from build123d import *

# Parameters (mm, degrees)
SKETCH1_R                = 5
BOSS_EXTRUDE1_DEPTH      = 120
SKETCH2_R                = 2.5
CUT_EXTRUDE1_DEPTH       = 20
SKETCH3_R                = 3
CUT_EXTRUDE2_DEPTH       = 80
SKETCH4_R                = 2
BOSS_EXTRUDE2_DEPTH      = 8
BOSS_EXTRUDE3_DEPTH      = 4
BOSS_EXTRUDE3_DEPTH_BACK = 4
SKETCH5_R                = 2.5
CUT_EXTRUDE3_DEPTH       = 121.208152802
CUT_EXTRUDE3_DEPTH_BACK  = 121.208152802
SKETCH6_R                = 2.5


with BuildPart() as part:
    # Sketch1 → Boss-Extrude1 (new body)
    with BuildSketch(Plane(origin=(0, 0, 0), x_dir=(0, 0, -1), z_dir=(1, 0, 0))):
        Circle(SKETCH1_R)
    extrude(amount=-BOSS_EXTRUDE1_DEPTH)

    # Sketch2 → Cut-Extrude1 (cut)
    with BuildSketch(Plane.ZY.offset(120)):
        Circle(SKETCH2_R)
    extrude(amount=-CUT_EXTRUDE1_DEPTH, mode=Mode.SUBTRACT)

    # Sketch3 → Cut-Extrude2 (cut)
    with BuildSketch(Plane.ZY.offset(100)):
        Circle(SKETCH3_R)
    extrude(amount=-CUT_EXTRUDE2_DEPTH, mode=Mode.SUBTRACT)

    # Sketch4 → Boss-Extrude2 (add)
    with BuildSketch(Plane(origin=(0, 0, 0), x_dir=(0, 0, -1), z_dir=(1, 0, 0))):
        Circle(SKETCH4_R)
    extrude(amount=BOSS_EXTRUDE2_DEPTH)

    # Sketch5 → Boss-Extrude3 (add, two sides: drawn at the far end of the back side and taken through both)
    with BuildSketch(Plane.XY.offset(-BOSS_EXTRUDE3_DEPTH_BACK)):
        with Locations((8, 0)):
            Circle(SKETCH5_R)
    extrude(amount=BOSS_EXTRUDE3_DEPTH + BOSS_EXTRUDE3_DEPTH_BACK)

    # Sketch6 → Cut-Extrude3 (cut, two sides: drawn at the far end of the back side and taken through both)
    with BuildSketch(Plane.XY.offset(-CUT_EXTRUDE3_DEPTH_BACK)):
        with Locations((-30, 0)):
            Circle(SKETCH6_R)
    extrude(amount=CUT_EXTRUDE3_DEPTH + CUT_EXTRUDE3_DEPTH_BACK, mode=Mode.SUBTRACT)


solid = part.part
Part model, mm, in its own coordinate system. A direction names the side the tool comes from. Coordinates: 2 decimals unless noted, no trailing zeros. Loops run counter-clockwise (first coordinate to the right, second up) from the corner with the lowest first, then second, coordinate; pieces in that order, holes last. Notation, with made-up numbers: M 42.25,-14 L 80.25,-14 A24 ccw 80.25,20 Z; hole C 47,78.5 d1. An arc over 180 degrees is marked long. Use a Markdown table: item, result. Add a question column.
Q1. Cut at A-A (y = 0). Write the cut outline in (x, z).
Q2. Mould opens along X. For faces 1 (the flat face through (8, 0, 4)), 2 (the flat face through (-120, -2, -2)), 3 (the cylindrical face through (3.204, -0.766, -1.847)) say: +X half, -X half, draft (parallel to the pull), parting line (faces both ways), or undercut.
Q3. Cut at D-D (x = -67). Write the cut outline in (y, z), and give its area (3 significant figures).
Q4. Cut at C-C (x = -30). Write the cut outline in (y, z).
Q5. Cut at B-B (z = 0). Write the cut outline in (x, y), and give its area (3 significant figures).
Q6. Which spindle directions (+Z, -Z, +X, -X, +Y, -Y) get a long thin tool onto all of the face, cutting with end or side? Do faces 4 (the cylindrical face through (-59.16, -4.88, 1.08)), 5 (the cylindrical face through (-27.69, -0.96, -3.35)), 6 (the cylindrical face through (-61, 0, -3)), 7 (the cylindrical face through (-110.14, -2.44, -0.54)), 8 (the flat face through (8, 0, -4)). Say none if no direction does.
Q7. Probe L1, parallel to X at y = -0.5, z = 3.25; L2, parallel to X at y = -2, z = 2.75; L3, parallel to Y at x = -67, z = 0. List the from-to ranges inside material, lowest first.
Q8. Pin check, flat tips, straight feed: P1, Ø1.5, axis at x = -86, z = -4, coming from the -Y side; P2, Ø6, axis at x = -27.5, y = 3.5, coming from the +Z side; P3, Ø1.5, axis at y = 1, z = -1.5, coming from the +X side. Stop position of each tip, or through.
Worked out:
| question | item | result |
|---|---|---|
| 1 | outline | M -120,-5 L -32.5,-5 L -32.5,-3 L -100,-3 L -100,-2.5 L -120,-2.5 Z; M -120,2.5 L -100,2.5 L -100,3 L -32.5,3 L -32.5,5 L -120,5 Z; M -27.5,-5 L 0,-5 L 0,-2 L 5.5,-2 L 5.5,-4 L 10.5,-4 L 10.5,4 L 5.5,4 L 5.5,2 L 0,2 L 0,5 L -27.5,5 L -27.5,3 L -20,3 L -20,-3 L -27.5,-3 Z |
| 2 | face 1 | draft |
| 2 | face 2 | -X half |
| 2 | face 3 | undercut |
| 3 | outline | C 0,0 d10; hole C 0,0 d6 |
| 3 | area | 50.3 mm2 |
| 4 | outline | M -2.5,-4.33 L -2.5,-1.66 A3 cw -2.5,1.66 L -2.5,4.33 A5 ccw Z; M 2.5,-4.33 A5 ccw 2.5,4.33 L 2.5,1.66 A3 cw 2.5,-1.66 Z |
| 5 | outline | M -120,-5 L 0,-5 L 0,-2 L 6.5,-2 A2.5 ccw long 6.5,2 L 0,2 L 0,5 L -120,5 L -120,2.5 L -100,2.5 L -100,3 L -20,3 L -20,-3 L -100,-3 L -100,-2.5 L -120,-2.5 Z |
| 5 | area | 663 mm2 |
| 6 | face 4 | +X, -X |
| 6 | face 5 | +Z, -Z |
| 6 | face 6 | none |
| 6 | face 7 | -X |
| 6 | face 8 | -Z, +X, +Y, -Y |
| 7 | L1 | x = -120 to -32.45, -27.55 to 0, 5.55 to 10.45 |
| 7 | L2 | x = -120 to -31.5, -28.5 to 0, 6.5 to 9.5 |
| 7 | L3 | y = -5 to -3, 3 to 5 |
| 8 | P1 | stops at y = -3.8 |
| 8 | P2 | stops at z = 4.97 |
| 8 | P3 | stops at x = 10.49 |
